Job drawing, mm, ordinate dimensions from the low corner. One solid piece. A direction names the side the tool comes from. Coordinates: 2 decimals unless noted, no trailing zeros. Write each loop counter-clockwise with the first axis right and the second up, starting at its lowest first coordinate (ties: lowest second). Pieces come first, ordered by that corner, then holes. Notation, with made-up numbers: (66, 80) - (76, 80) arc R27 ccw to (76, 116) - close; hole circle Ø2 at (-32.5, 77). An arc over 180 degrees is marked (long way). Use a Markdown table: item, result.
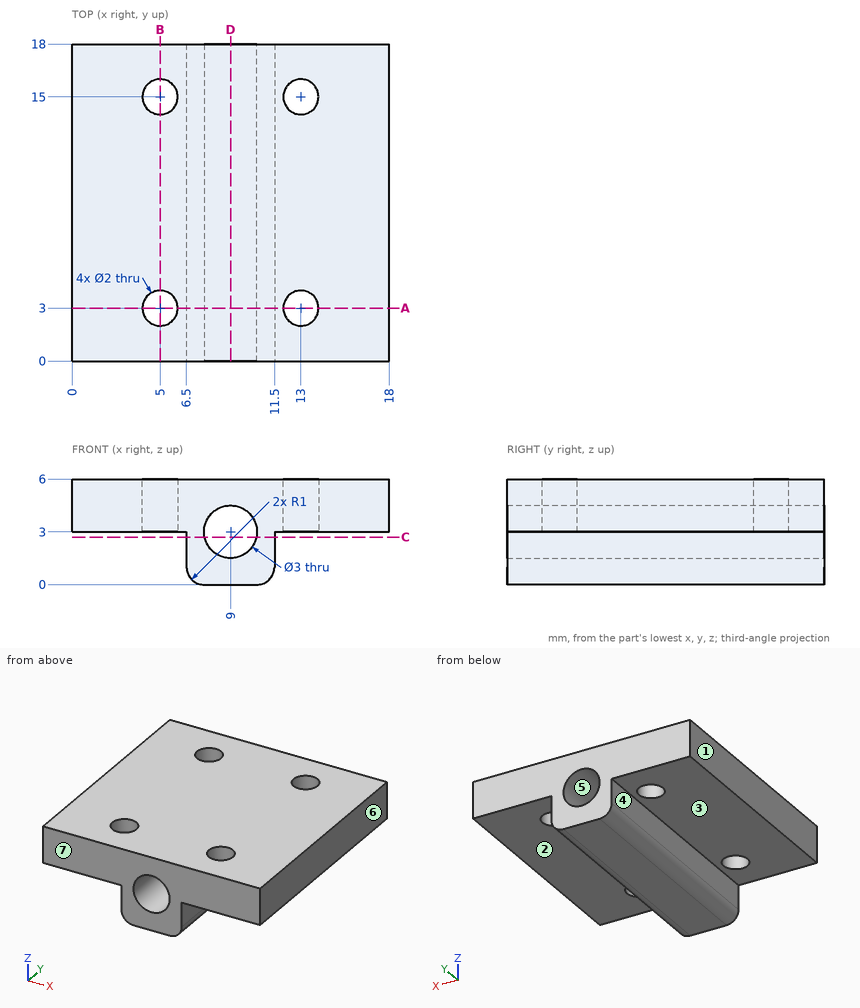
Item 1: Which spindle directions (+Z, -Z, +X, -X, +Y, -Y) get a long thin tool onto all of the face, cutting with end or side? Do the marked faces 1, 2 and 3. Say none if no direction does.
From the geometry:
| item | result |
|---|---|
| face 1 | +Z, -Z, -X, +Y, -Y |
| face 2 | -Z, +X, +Y, -Y |
| face 3 | -Z, -X, +Y, -Y |
Item 2: Band-saw the part on A-A, the plane y = 3. Give the cut face in (x, z), then the cut area to 3 significant figures.
From the geometry:
| item | result |
|---|---|
| outline | (0, 3) - (4, 3) - (4, 6) - (0, 6) - close; (6, 3) - (6.5, 3) - (6.5, 1) arc R1 ccw to (7.5, 0) - (10.5, 0) arc R1 ccw to (11.5, 1) - (11.5, 3) - (12, 3) - (12, 6) - (6, 6) - close; (14, 3) - (18, 3) - (18, 6) - (14, 6) - close; hole circle Ø3 at (9, 3) |
| area | 49.5 mm^2 |
Item 3: Band-saw the part on D-D, the plane x = 9. Give the cut face in (y, z), then the cut area to 3 significant figures.
From the geometry:
| item | result |
|---|---|
| outline | (0, 0) - (18, 0) - (18, 1.5) - (0, 1.5) - close; (0, 4.5) - (18, 4.5) - (18, 6) - (0, 6) - close |
| area | 54.0 mm^2 |
Item 4: Band-saw the part on B-B, the plane x = 5. Give the cut face in (y, z), then the cut area to 3 significant figures.
From the geometry:
| item | result |
|---|---|
| outline | (0, 3) - (2, 3) - (2, 6) - (0, 6) - close; (4, 3) - (14, 3) - (14, 6) - (4, 6) - close; (16, 3) - (18, 3) - (18, 6) - (16, 6) - close |
| area | 42.0 mm^2 |
Item 5: Two-plate mould, pull along X, no slides. Class the marked faces 4, 5, 6 and 7: pulls with the +X half, pulls with the -X half, needs draft (parallel to the pull), parting line crosses it, or undercut.
From the geometry:
| item | result |
|---|---|
| face 4 | pulls with the -X half |
| face 5 | undercut |
| face 6 | pulls with the +X half |
| face 7 | needs draft |
Item 6: Drill centre lines: probe 1 along Y at (x, z) = (13, 4.3); probe 2 along Z at (x, y) = (9, 9.5); probe 3 along Z at (x, y) = (2, 11). Where is each one in solid material? Low to high.
From the geometry:
| item | result |
|---|---|
| probe 1 | 0 to 2, 4 to 14, 16 to 18 |
| probe 2 | 0 to 1.5, 4.5 to 6 |
| probe 3 | 3 to 6 |
Item 7: Drop flat-ended pins along their axis: P1, Ø7, axis at x = 3.5, y = 5.5, coming from the -Z side; P2, Ø2, axis at y = 11, z = 1.5, coming from the -X side. Give the stop position or say it passes through.
From the geometry:
| item | result |
|---|---|
| P1 | z = 0.13 |
| P2 | x = 6.5 |
Item 8: Band-saw the part on C-C, the plane z = 2.7. Give the cut face in (x, y), then the cut area to 3 significant figures.
From the geometry:
| item | result |
|---|---|
| outline | (6.5, 0) - (7.53, 0) - (7.53, 18) - (6.5, 18) - close; (10.47, 0) - (11.5, 0) - (11.5, 18) - (10.47, 18) - close |
| area | 37.1 mm^2 |
